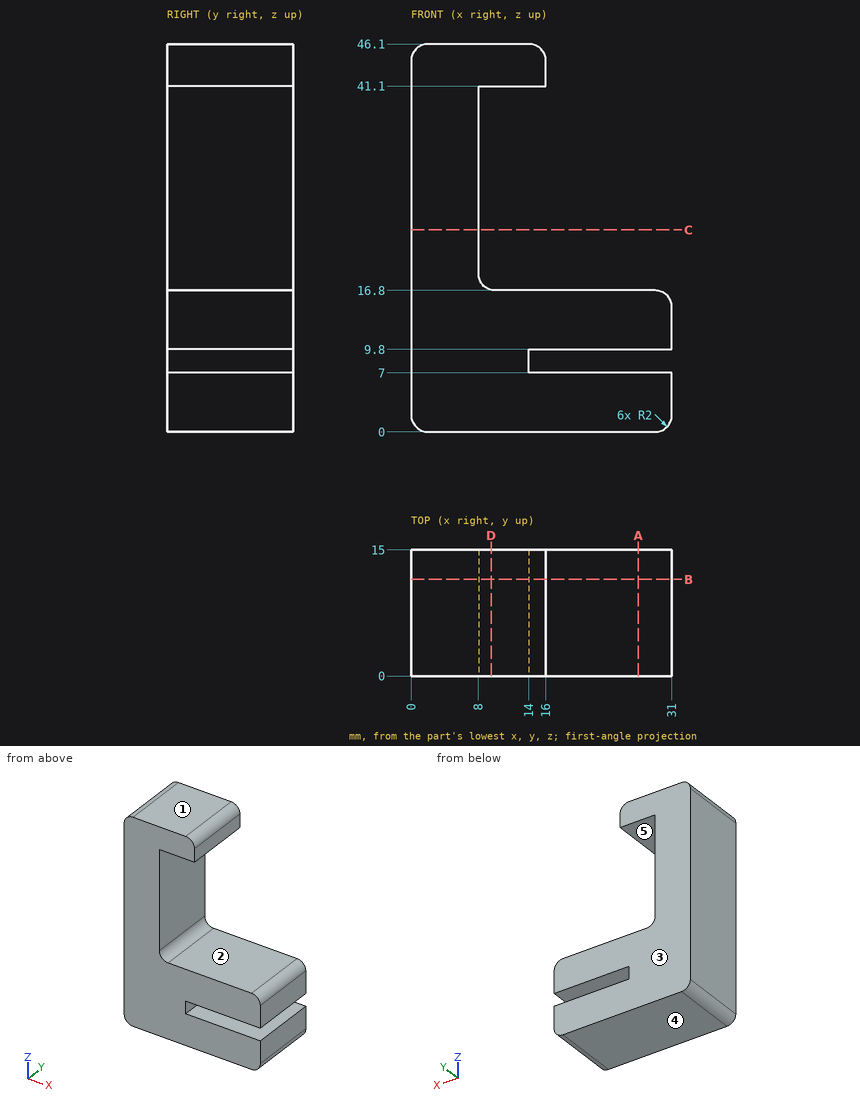
Source: three-view drawing plus pictorial views. Frame: mm from the lowest corner of the part. A direction names the side the tool comes from. Give positions to 0.01 mm unless a question says otherwise; leave off trailing zeros. Write each loop counter-clockwise with the first axis right and the second up, starting at its lowest first coordinate (ties: lowest second). Pieces come first, ordered by that corner, then holes.
(1) Cut plane C-C, the plane z = 24. Return loops of the section in (x, y), then the cut area to 3 significant figures.
(2) Mould query, pull axis Z, two halves, no side actions, for the marked faces 1, 2 and 3. Classes: released by +Z, released by -Z, zero draft, split by the parting line, or undercut.
(3) Cut plane A-A, the plane x = 27. Return loops of the section in (y, z).
(4) Cut plane D-D, the plane x = 9.5. Return loops of the section in (y, z).
(5) Ray query, line 1 (Z direction, x = 21.5, y = 10.5); line 2 (X direction, y = 2.75, z = 39); line 3 (X direction, y = 1, z = 42.5). Return the intervals inside material, ascending.
(6) Access query for the marked faces 4 and 5. Directions: +Z, -Z, +X, -X, +Y, -Y. A direction counts if a zero-diameter tool reaches every point of the face in a straight line with its end or side. Return the directions, or none.
(7) Cut plane B-B, the plane y = 11.5. Return loops of the section in (x, z).
(8) First-contact query: P1, Ø0.8, axis at y = 7, z = 9, coming from the +X side; P2, Ø8, axis at x = 3.5, z = 13, coming from the -Y side; P3, Ø3.5, axis at y = 6.5, z = 43, coming from the +X side; P4, Ø7.5, axis at x = 21, y = 6, coming from the +Z side. Flat tips, straight axial feed; report the tip coordinate or a pass-through.
Values follow:
1. outline: (0, 0) - (8, 0) - (8, 15) - (0, 15) - close
1. area: 120 mm2
2. face 1: released by +Z
2. face 2: undercut
2. face 3: zero draft
3. outline: (0, 0) - (15, 0) - (15, 7) - (0, 7) - close; (0, 9.8) - (15, 9.8) - (15, 16.8) - (0, 16.8) - close
4. outline: (0, 0) - (15, 0) - (15, 16.86) - (0, 16.86) - close; (0, 41.1) - (15, 41.1) - (15, 46.1) - (0, 46.1) - close
5. line 1: z = 0 to 7, 9.8 to 16.8
5. line 2: x = 0 to 8
5. line 3: x = 0 to 16
6. face 4: -Z, +X, -X, +Y, -Y
6. face 5: +X, +Y, -Y
7. outline: (0, 2) arc R2 ccw to (2, 0) - (29, 0) arc R2 ccw to (31, 2) - (31, 7) - (14, 7) - (14, 9.8) - (31, 9.8) - (31, 14.8) arc R2 ccw to (29, 16.8) - (10, 16.8) arc R2 cw to (8, 18.8) - (8, 41.1) - (16, 41.1) - (16, 44.1) arc R2 ccw to (14, 46.1) - (2, 46.1) arc R2 ccw to (0, 44.1) - close
8. P1: stops at x = 14
8. P2: stops at y = 0
8. P3: stops at x = 16
8. P4: stops at z = 16.8
